```python
from build123d import *

# Parameters (mm, degrees)
SKETCH_1_W          = 100
SKETCH_1_H          = 65
EXTRUDE_1_DEPTH     = 12
SKETCH_2_R          = 3.5
CUT_EXTRUDE_1_DEPTH = 61.829680256
SKETCH_3_R          = 1.5
CUT_EXTRUDE_2_DEPTH = 10
CUT_EXTRUDE_START   = -10
SKETCH_4_R          = 1.5
CUT_EXTRUDE_3_DEPTH = 10
FILLET_1_R          = 2


with BuildPart() as part:
    # 草图1 → 凸台-拉伸1 (new body)
    with BuildSketch(Plane.XY):
        Rectangle(SKETCH_1_W, SKETCH_1_H)
    extrude(amount=EXTRUDE_1_DEPTH)

    # 草图2 → 切除-拉伸1 (cut, through all)
    with BuildSketch(Plane.XY.offset(12)):
        with Locations((-40, -9)):
            Circle(SKETCH_2_R)
        with Locations((40, -9)):
            Circle(SKETCH_2_R)
        with BuildLine():
            Line((30, 31), (-30, 31))
            ThreePointArc((-30, 31), (-30.632455532, 30.897366596), (-31.2, 30.6))
            Line((-31.2, 30.6), (-32.8, 29.4))
            ThreePointArc((-32.8, 29.4), (-33.367544468, 29.102633404), (-34, 29))
            Line((-34, 29), (-41, 29))
            ThreePointArc((-41, 29), (-43.828427125, 27.828427125), (-45, 25))
            Line((-45, 25), (-45, 4.964240044))
            ThreePointArc((-45, 4.964240044), (-43.725540575, 2.036539825), (-40.714285714, 0.974457174))
            ThreePointArc((-40.714285714, 0.974457174), (-30.006387747, -8.642628863), (-40, -19))
            ThreePointArc((-40, -19), (-45, -24), (-40, -29))
            Line((-40, -29), (-34, -29))
            ThreePointArc((-34, -29), (-33.367544468, -29.102633404), (-32.8, -29.4))
            Line((-32.8, -29.4), (-31.2, -30.6))
            ThreePointArc((-31.2, -30.6), (-30.632455532, -30.897366596), (-30, -31))
            Line((-30, -31), (30, -31))
            ThreePointArc((30, -31), (30.632455532, -30.897366596), (31.2, -30.6))
            Line((31.2, -30.6), (32.8, -29.4))
            ThreePointArc((32.8, -29.4), (33.367544468, -29.102633404), (34, -29))
            Line((34, -29), (40, -29))
            ThreePointArc((40, -29), (45, -24), (40, -19))
            ThreePointArc((40, -19), (30.006387747, -8.642628863), (40.714285714, 0.974457174))
            ThreePointArc((40.714285714, 0.974457174), (43.725540575, 2.036539825), (45, 4.964240044))
            Line((45, 4.964240044), (45, 25))
            ThreePointArc((45, 25), (43.828427125, 27.828427125), (41, 29))
            Line((41, 29), (34, 29))
            ThreePointArc((34, 29), (33.367544468, 29.102633404), (32.8, 29.4))
            Line((32.8, 29.4), (31.2, 30.6))
            ThreePointArc((31.2, 30.6), (30.632455532, 30.897366596), (30, 31))
        make_face()
    extrude(amount=-CUT_EXTRUDE_1_DEPTH, mode=Mode.SUBTRACT)

    # 草图3 → 切除-拉伸2 (cut)
    with BuildSketch(Plane(origin=(0, 32.5, 0), x_dir=(1, 0, 0), z_dir=(0, 1, 0))):
        with Locations(Location((40, -6, 0), (0, 0, 270))):
            Circle(SKETCH_3_R)
    cut_extrude_2 = extrude(amount=-CUT_EXTRUDE_2_DEPTH, mode=Mode.SUBTRACT)

    # 草图4 → 切除-拉伸3 (cut)
    with BuildSketch(Plane.XZ.offset(32.5).offset(CUT_EXTRUDE_START)):
        with Locations(Location((40, 6, 0), (0, 0, 90))):
            Circle(SKETCH_4_R)
    cut_extrude_3 = extrude(amount=CUT_EXTRUDE_3_DEPTH, mode=Mode.SUBTRACT)

    # 镜向1: 切除-拉伸2, 切除-拉伸3 across plane
    add(cut_extrude_2.mirror(Plane(origin=(0, 0, 0), x_dir=(0, 0, 1), z_dir=(1, 0, 0))), mode=Mode.SUBTRACT)
    add(cut_extrude_3.mirror(Plane(origin=(0, 0, 0), x_dir=(0, 0, 1), z_dir=(1, 0, 0))), mode=Mode.SUBTRACT)

    # 圆角1
    fillet_1_edges = [part.edges().sort_by_distance(p)[0] for p in [
        (-50, 0, 12),
        (50, 0, 12),
    ]]
    fillet(fillet_1_edges, radius=FILLET_1_R)


solid = part.part
```
Could you check a few things on this model? Use its own coordinates, in mm. A direction names the side the tool comes from. Coordinates: 2 decimals unless noted, no trailing zeros. Loops run counter-clockwise (first coordinate to the right, second up) from the corner with the lowest first, then second, coordinate; pieces in that order, holes last.
1) Imagine slicing it at A-A (y = -24). List the corners of the cut face in (x, z) for me.
Reported:
outline: (-50, 0) - (-45, 0) - (-45, 12) - (-48, 12) arc R2 ccw to (-50, 10) - close; (45, 0) - (50, 0) - (50, 10) arc R2 ccw to (48, 12) - (45, 12) - close
2) Which directions (+Z, -Z, +X, -X, +Y, -Y) give clear straight access to the entire face, cutting with the end or side of a thin tool? Please do faces 5 (the face through (-49.43, 0.45, 11.4)), 6 (the face through (-38.536, 30.759, 5.675)), 7 (the face through (41.464, -30.609, 5.675)), 8 (the face through (43.859, 27.797, 6.084)), 9 (the face through (-1, 32.5, 6)).
Reported:
face 5: +Z, -X, +Y, -Y
face 6: +Y
face 7: -Y
face 8: +Z, -Z
face 9: +Z, -Z, +X, -X, +Y
3) Will these pins go through, and if not, where does the flat tip stop? pin 1 Ø1.8 at (x, z) = (40, 6) entering from -Y; pin 2 Ø11 at (x, y) = (40, -9) entering from -Z.
Reported:
pin 1: stops at y = -19.08
pin 2: stops at z = 0
4) Please list where these lines run through material, in increasing order: line 1 along Y through (x, z) = (9, 1); line 2 along Y through (x, z) = (-40, 4.25); line 3 along Z through (x, y) = (-40, 30.25).
Reported:
line 1: y = -32.5 to -31, 31 to 32.5
line 2: y = -32.5 to -29, -19 to -12.5, -5.5 to 1, 29 to 32.5
line 3: z = 0 to 4.5, 7.5 to 12
5) Imagine slicing it at B-B (x = 25.5). List the corners of the cut face in (y, z) for me, and give its area (3 significant figures).
Reported:
outline: (-32.5, 0) - (-31, 0) - (-31, 12) - (-32.5, 12) - close; (31, 0) - (32.5, 0) - (32.5, 12) - (31, 12) - close
area: 36.0 mm2
6) Imagine slicing it at D-D (x = -37.5). List the corners of the cut face in (y, z) for me, and give its area (3 significant figures).
Reported:
outline: (-32.5, 0) - (-29, 0) - (-29, 12) - (-32.5, 12) - close; (-18.68, 0) - (-11.45, 0) - (-11.45, 12) - (-18.68, 12) - close; (-6.55, 0) - (0.68, 0) - (0.68, 12) - (-6.55, 12) - close; (29, 0) - (32.5, 0) - (32.5, 12) - (29, 12) - close
area: 258 mm2
7) Thinking about a two-plate mould opening in X: for faces 1 (the face through (-1, -32.5, 6)), 2 (the face through (-37, 29, 6)), 3 (the face through (50, 0, 5)), 4 (the face through (-50, 0, 5)), which applies, released by +X, released by -X, zero draft, split by the parting line, or undercut?
Reported:
face 1: zero draft
face 2: undercut
face 3: released by +X
face 4: released by -X
8) Imagine slicing it at C-C (y = -9). List the corners of the cut face in (x, z) for me, and give its area (3 significant figures).
Reported:
outline: (-50, 0) - (-43.5, 0) - (-43.5, 12) - (-48, 12) arc R2 ccw to (-50, 10) - close; (-36.5, 0) - (-30, 0) - (-30, 12) - (-36.5, 12) - close; (30, 0) - (36.5, 0) - (36.5, 12) - (30, 12) - close; (43.5, 0) - (50, 0) - (50, 10) arc R2 ccw to (48, 12) - (43.5, 12) - close
area: 310 mm2
